from build123d import *

# Parameters (mm, degrees)
F0_R     = 3.1
F0_R_2   = 56.75
F0_R_3   = 4.1
F1_DEPTH = 6


with BuildPart() as f1:
    # F0 (on Right) → F1 (new body)
    with BuildSketch(Plane.YZ):
        with BuildLine():
            Line((-220, 0), (-20, 0))
            ThreePointArc((-20, 0), (-5.857864, 5.857864), (0, 20))
            Line((0, 20), (0, 187.857864))
            ThreePointArc((0, 187.857864), (-0.761205, 191.684699), (-2.928932, 194.928932))
            Line((-2.928932, 194.928932), (-37.071068, 229.071068))
            ThreePointArc((-37.071068, 229.071068), (-40.315301, 231.238795), (-44.142136, 232))
            Line((-44.142136, 232), (-50, 232))
            Line((-50, 232), (-50, 217))
            Line((-50, 217), (-124.666667, 161))
            ThreePointArc((-124.666667, 161), (-130.342111, 158.026334), (-136.666667, 157))
            Line((-136.666667, 157), (-155, 157))
            ThreePointArc((-155, 157), (-200.961941, 137.961941), (-220, 92))
            Line((-220, 92), (-220, 0))
        make_face()
        with Locations((-177.25, 29.141361)):
            Circle(F0_R, mode=Mode.SUBTRACT)
        with Locations((-112.75, 29.141361)):
            Circle(F0_R, mode=Mode.SUBTRACT)
        with Locations((-209.5, 85)):
            Circle(F0_R, mode=Mode.SUBTRACT)
        with Locations((-145, 85)):
            Circle(F0_R_2, mode=Mode.SUBTRACT)
        with Locations((-72.986513, 29.659025)):
            Circle(F0_R_3, mode=Mode.SUBTRACT)
        with Locations((-25, 15.477134)):
            Circle(F0_R_3, mode=Mode.SUBTRACT)
        with Locations((-25, 43.423373)):
            Circle(F0_R_3, mode=Mode.SUBTRACT)
        with Locations((-80.5, 85)):
            Circle(F0_R, mode=Mode.SUBTRACT)
        with Locations((-25, 69.423373)):
            Circle(F0_R_3, mode=Mode.SUBTRACT)
        with Locations((-25, 95.423373)):
            Circle(F0_R_3, mode=Mode.SUBTRACT)
        with Locations((-177.25, 140.858639)):
            Circle(F0_R, mode=Mode.SUBTRACT)
        with Locations((-112.75, 140.858639)):
            Circle(F0_R, mode=Mode.SUBTRACT)
        with Locations((-63.867599, 127.938718)):
            Circle(F0_R_3, mode=Mode.SUBTRACT)
        with Locations((-90.302517, 168.023112)):
            Circle(F0_R_3, mode=Mode.SUBTRACT)
        with Locations((-68.746537, 162.530556)):
            Circle(F0_R_3, mode=Mode.SUBTRACT)
        with Locations((-25, 121.423373)):
            Circle(F0_R_3, mode=Mode.SUBTRACT)
        with Locations((-25, 147.423373)):
            Circle(F0_R_3, mode=Mode.SUBTRACT)
        with Locations((-25, 173.423373)):
            Circle(F0_R_3, mode=Mode.SUBTRACT)
        with Locations((-74.302517, 180.023112)):
            Circle(F0_R_3, mode=Mode.SUBTRACT)
        with Locations((-58.302517, 192.023112)):
            Circle(F0_R_3, mode=Mode.SUBTRACT)
        with Locations((-25, 199.423373)):
            Circle(F0_R_3, mode=Mode.SUBTRACT)
    extrude(amount=F1_DEPTH)


solid = f1.part
Verification items for the finished model (mm, model axes). A direction names the side the tool comes from. Coordinates: 2 decimals unless noted, no trailing zeros. Write each loop counter-clockwise with the first axis right and the second up, starting at its lowest first coordinate (ties: lowest second). Pieces come first, ordered by that corner, then holes. Notation, with made-up numbers: M 73.25,48.25 L 109.25,48.25 A14 ccw 109.25,53.25 Z; hole C 82,58.5 d2. An arc over 180 degrees is marked long. Use a Markdown table: item, result.
Q1. Draft check along Z on faces 3 (the face through (2.96, -67.12, 125.44)), 4 (the face through (3, -121, 0)), 5 (the face through (3, -220, 47)). Enter one of: +Z half, -Z half, draft (parallel to the pull), parting line (faces both ways), or undercut.
Reply:
| item | result |
|---|---|
| face 3 | undercut |
| face 4 | -Z half |
| face 5 | draft |
Q2. Set-up check for faces 1 (the face through (2.96, -59.19, 188.02)), 2 (the face through (3, -50, 225)): record each of +Z, -Z, +X, -X, +Y, -Y from which the full face is reachable in a straight line by a thin tool's end or side.
Reply:
| item | result |
|---|---|
| face 1 | +X, -X |
| face 2 | +Z, +X, -X, -Y |
Q3. Sectioned sample at B-B, the plane y = -177.25. Record the boundary of the cut face in (x, z).
Reply:
| item | result |
|---|---|
| outline | M 0,0 L 6,0 L 6,26.04 L 0,26.04 Z; M 0,32.24 L 6,32.24 L 6,38.3 L 0,38.3 Z; M 0,131.7 L 6,131.7 L 6,137.76 L 0,137.76 Z; M 0,143.96 L 6,143.96 L 6,153.07 L 0,153.07 Z |
Q4. Sectioned sample at A-A, the plane z = 85. Record the boundary of the cut face in (x, y).
Reply:
| item | result |
|---|---|
| outline | M 0,-220 L 6,-220 L 6,-212.6 L 0,-212.6 Z; M 0,-206.4 L 6,-206.4 L 6,-201.75 L 0,-201.75 Z; M 0,-88.25 L 6,-88.25 L 6,-83.6 L 0,-83.6 Z; M 0,-77.4 L 6,-77.4 L 6,0 L 0,0 Z |
Q5. Sectioned sample at C-C, the plane x = 2.25. Count the separate pieces of the cut face and the enclosed holes in it, plus the area to 3 significant figures.
Reply:
| item | result |
|---|---|
| separate pieces | 1 |
| enclosed holes | 21 |
| area | 27,900 mm² |
Q6. Thickness scan on line 1 (Z direction, x = 2.9, y = -145); line 2 (Y direction, x = 4.55, z = 125); line 3 (Z direction, x = 5.3, y = -112). Record the ranges inside material, lowest first.
Reply:
| item | result |
|---|---|
| line 1 | z = 0 to 28.25, 141.75 to 157 |
| line 2 | y = -211 to -185.26, -104.74 to -66.73, -61.01 to -27, -23 to 0 |
| line 3 | z = 0 to 26.13, 32.15 to 38.83, 131.17 to 137.85, 143.87 to 170.5 |
Q7. Go/stop test with flat-tipped pins: P1, Ø1.5, axis at x = 4, y = -125.5, coming from the +Z side; P2, Ø3, axis at x = 2.5, y = -147.5, coming from the +Z side. Record where each tip stops, or that it passes through.
Reply:
| item | result |
|---|---|
| P1 | stops at z = 160.94 |
| P2 | stops at z = 157 |
